```python
from build123d import *

# Parameters (mm, degrees)
CYLINDER001_R       = 4
CYLINDER001_DEPTH   = 10
CYLINDER_R          = 8
CYLINDER_DEPTH      = 7
CUT_PITCH_ANGLE     = 90
CUT_PLACEMENT_ANGLE = 90
SKETCH_W            = 80
SKETCH_H            = 52
SKETCH_R            = 2.1
PAD_DEPTH           = 10
SKETCH009_R         = 11.15
PAD001_DEPTH        = 9
SKETCH010_R         = 3.6
POCKET_DEPTH        = 2.4


with BuildPart() as zylinder001:
    # Cylinder001 → Cylinder001 (new body)
    with BuildSketch(Plane.XY):
        Circle(CYLINDER001_R)
    extrude(amount=CYLINDER001_DEPTH)


with BuildPart() as cut:
    # Cylinder → Cylinder (new body)
    with BuildSketch(Plane.XY):
        Circle(CYLINDER_R)
    extrude(amount=CYLINDER_DEPTH)

    # Cut: cut Zylinder001
    add(zylinder001.part, mode=Mode.SUBTRACT)


with BuildPart() as cut_1:
    # Cut pitch: moved
    add(cut.part.rotate(Axis((0, 0, 0), (0, 1, 0)), CUT_PITCH_ANGLE))


with BuildPart() as cut_2:
    # Cut placement: moved
    add(cut_1.part.moved(Location((-14, 0, 7))).rotate(Axis((-14, 0, 7), (0, 0, 1)), CUT_PLACEMENT_ANGLE))


with BuildPart() as pocket:
    # Sketch → Pad (new body)
    with BuildSketch(Plane.XY):
        Rectangle(SKETCH_W, SKETCH_H)
        with Locations((-30, -16)):
            Circle(SKETCH_R, mode=Mode.SUBTRACT)
        with Locations((-30, 4)):
            Circle(SKETCH_R, mode=Mode.SUBTRACT)
        with Locations((30, 4)):
            Circle(SKETCH_R, mode=Mode.SUBTRACT)
        with Locations((30, -16)):
            Circle(SKETCH_R, mode=Mode.SUBTRACT)
    extrude(amount=PAD_DEPTH)

    # Sketch009 → Pad001 (new body)
    with BuildSketch(Plane(origin=(0, 26, 0), x_dir=(-1, 0, 0), z_dir=(0, 1, 0))):
        with BuildLine():
            ThreePointArc((21.15, 31.150033), (-1.7e-05, 52.3), (-21.15, 31.15))
            Line((-21.15, 31.15), (-21.15, 10))
            Line((-21.15, 10), (21.15, 10))
            Line((21.15, 10), (21.15, 31.150033))
        make_face()
        with Locations((0, 31.15)):
            Circle(SKETCH009_R, mode=Mode.SUBTRACT)
    extrude(amount=-PAD001_DEPTH)

    # Cut001: cut Cut
    add(cut_2.part, mode=Mode.SUBTRACT)

    # Sketch010 → Pocket (cut)
    with BuildSketch(Plane.XY.offset(10)):
        with Locations((-30, 4)):
            Circle(SKETCH010_R)
        with Locations((-30, -16)):
            Circle(SKETCH010_R)
        with Locations((30, -16)):
            Circle(SKETCH010_R)
        with Locations((30, 4)):
            Circle(SKETCH010_R)
    extrude(amount=-POCKET_DEPTH, mode=Mode.SUBTRACT)


solid = pocket.part
```
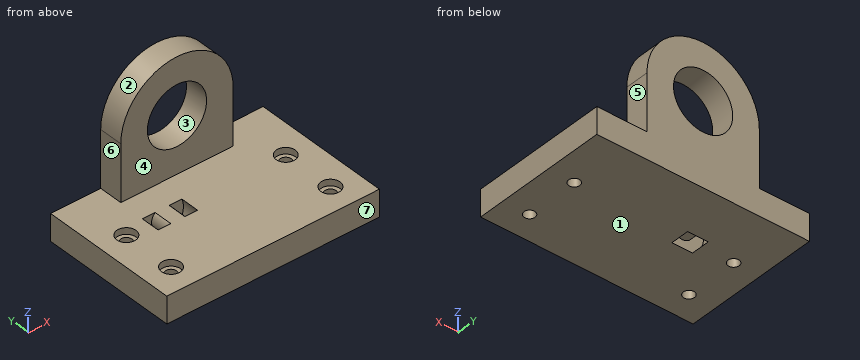
Can you work these out from the model? Positions are in its coordinate system, mm. Face numbers are marked on the shaded views. A direction names the side the tool comes from. Coordinates: 2 decimals unless noted, no trailing zeros. Order: outer loops, then holes, each group sorted by start corner. A loop starts at its lowest first (then second) coordinate and runs counter-clockwise, first axis right, second up.
1. I need wall thicknesses on line 1 (Y direction, x = -30, z = 9.3); line 2 (Y direction, x = 30, z = 4.25); line 3 (X direction, y = -16, z = 2.25). Which ranges of each line are inside material? Lowest first, please.
2. If we section it at B-B (y = 20.5): Please give me the cut outline in (x, z).
3. I'm going to push flat-ended pins straight in: pin 1 (3.5 mm diameter, centred on x = 29, y = 3.5, fed in from +Z); pin 2 (11.5 mm diameter, centred on x = 30, y = -16, fed in from +Z); pin 3 (10 mm diameter, centred on y = 21, z = 19, fed in from +X). Where does each tip first touch, or does it pass through?
4. If we section it at A-A (x = 30): Please give me the cut outline in (y, z), then the cut area to 3 significant figures.
5. If we section it at C-C (y = -16): Please give me the cut outline in (x, z), then the cut area to 3 significant figures.
6. Thinking about a two-plate mould opening in Z: for the marked faces 1, 2, 3 and 4, which applies, +Z half, -Z half, draft (parallel to the pull), parting line (faces both ways), or undercut?
7. If we section it at D-D (z = 28): Please give me the cut outline in (x, y), then the cut area to 3 significant figures.
8. For the marked faces 5, 6 and 7, which set-ups out of +Z, -Z, +X, -X, +Y, -Y let a thin tool reach every point of the face, with its end or its side?
Entries:
1. line 1: y = -26 to -19.6, -12.4 to 0.4, 7.6 to 26
1. line 2: y = -26 to -18.1, -13.9 to 1.9, 6.1 to 26
1. line 3: x = -40 to -32.1, -27.9 to 27.9, 32.1 to 40
2. outline: (-40, 0) - (40, 0) - (40, 10) - (21.15, 10) - (21.15, 31.15) arc R21.15 ccw to (-21.15, 31.15) - (-21.15, 10) - (-40, 10) - close; hole circle Ø22.3 at (0, 31.15)
3. pin 1: stops at z = 7.6
3. pin 2: stops at z = 10
3. pin 3: stops at x = 21.15
4. outline: (-26, 0) - (-18.1, 0) - (-18.1, 7.6) - (-19.6, 7.6) - (-19.6, 10) - (-26, 10) - close; (-13.9, 0) - (1.9, 0) - (1.9, 7.6) - (0.4, 7.6) - (0.4, 10) - (-12.4, 10) - (-12.4, 7.6) - (-13.9, 7.6) - close; (6.1, 0) - (26, 0) - (26, 10) - (7.6, 10) - (7.6, 7.6) - (6.1, 7.6) - close
4. area: 422 mm2
5. outline: (-40, 0) - (-32.1, 0) - (-32.1, 7.6) - (-33.6, 7.6) - (-33.6, 10) - (-40, 10) - close; (-27.9, 0) - (27.9, 0) - (27.9, 7.6) - (26.4, 7.6) - (26.4, 10) - (-26.4, 10) - (-26.4, 7.6) - (-27.9, 7.6) - close; (32.1, 0) - (40, 0) - (40, 10) - (33.6, 10) - (33.6, 7.6) - (32.1, 7.6) - close
5. area: 702 mm2
6. face 1: -Z half
6. face 2: +Z half
6. face 3: undercut
6. face 4: draft
7. outline: (-21.15, 17) - (-10.7, 17) - (-10.7, 26) - (-21.15, 26) - close; (10.7, 17) - (21.15, 17) - (21.15, 26) - (10.7, 26) - close
7. area: 188 mm2
8. face 5: +Z, +X, +Y, -Y
8. face 6: +Z, -X, +Y, -Y
8. face 7: +Z, -Z, +X, -X, -Y
